from build123d import *

# Parameters (mm, degrees)
F0_R     = 3.15
F1_DEPTH = 5
F2_R     = 1


with BuildPart() as f1:
    # F0 (on Top) → F1 (new body)
    with BuildSketch(Plane.XY):
        with BuildLine():
            Line((-8, 7), (-7.482267, -0.515448))
            ThreePointArc((-7.482267, -0.515448), (0, -7.5), (7.482267, -0.515448))
            Line((7.482267, -0.515448), (8, 7))
            ThreePointArc((8, 7), (0, 9.5), (-8, 7))
        make_face()
        Circle(F0_R, mode=Mode.SUBTRACT)
    extrude(amount=F1_DEPTH)

    # F2
    f2_edges = [f1.edges().sort_by_distance(p)[0] for p in [
        (-8, 7, 2.5),
        (0, -7.5, 5),
        (0, 9.5, 5),
        (8, 7, 2.5),
        (-3.15, 0, 5),
    ]]
    fillet(f2_edges, radius=F2_R)


solid = f1.part
Work out the finished part from the listing and answer in its coordinate system (mm). Round coordinates to 2 decimals unless told otherwise and drop trailing zeros. Order: outer loops, then holes, each group sorted by start corner. A loop starts at its lowest first (then second) coordinate and runs counter-clockwise, first axis right, second up. Notation, with made-up numbers: M 34,85 L 59,85 A25 ccw 59,110 Z; hole C 22.5,6 d7. An arc over 180 degrees is marked long. One line per item, written item: value.
Q1. Determine the mould class of faces 1 (the face through (-2.5, -1.917, 1.972)), 2 (the face through (7.718, 2.903, 1.972)), 3 (the face through (-0.1, 4.4, 5)) for opening direction Y: released by +Y, released by -Y, zero draft, split by the parting line, or undercut.
Derived:
face 1: undercut
face 2: released by -Y
face 3: zero draft
Q2. Find section B-B on z = 1.6. Write down the section's boundary in (x, y), then the cut area to 3 significant figures.
Derived:
outline: M -7.96,6.42 L -7.48,-0.52 A7.5 ccw 7.48,-0.52 L 7.96,6.42 A1 ccw 7.5,7.33 A14.05 ccw -7.5,7.33 A1 ccw Z; hole C 0,0 d6.3
area: 193 mm²
Q3. Straight lines are drawn through the part: line 1 (X direction, y = 2.25, z = 2); line 2 (X direction, y = -1.5, z = 1.05); line 3 (Y direction, x = 1, z = 1.5). For each, find the intervals that lie inside material, in ascending order.
Derived:
line 1: -7.67 to -2.2, 2.2 to 7.67
line 2: -7.35 to -2.77, 2.77 to 7.35
line 3: -7.43 to -2.99, 2.99 to 9.46
Q4. Find section A-A on x = 0. Write down the section's boundary in (y, z).
Derived:
outline: M -7.5,0 L -3.15,0 L -3.15,4 A1 ccw -4.15,5 L -6.5,5 A1 ccw -7.5,4 Z; M 3.15,0 L 9.5,0 L 9.5,4 A1 ccw 8.5,5 L 4.15,5 A1 ccw 3.15,4 Z
Q5. Flat-ended cylindrical pins translate along their axes: pin 1 (3 mm diameter, centred on y = 7, z = 3.5, fed in from +X); pin 2 (5 mm diameter, centred on x = 0, y = 0, fed in from -Z). Find the tip coordinate at first contact, or state that the pin passes through.
Derived:
pin 1: x = 7.96
pin 2: through
